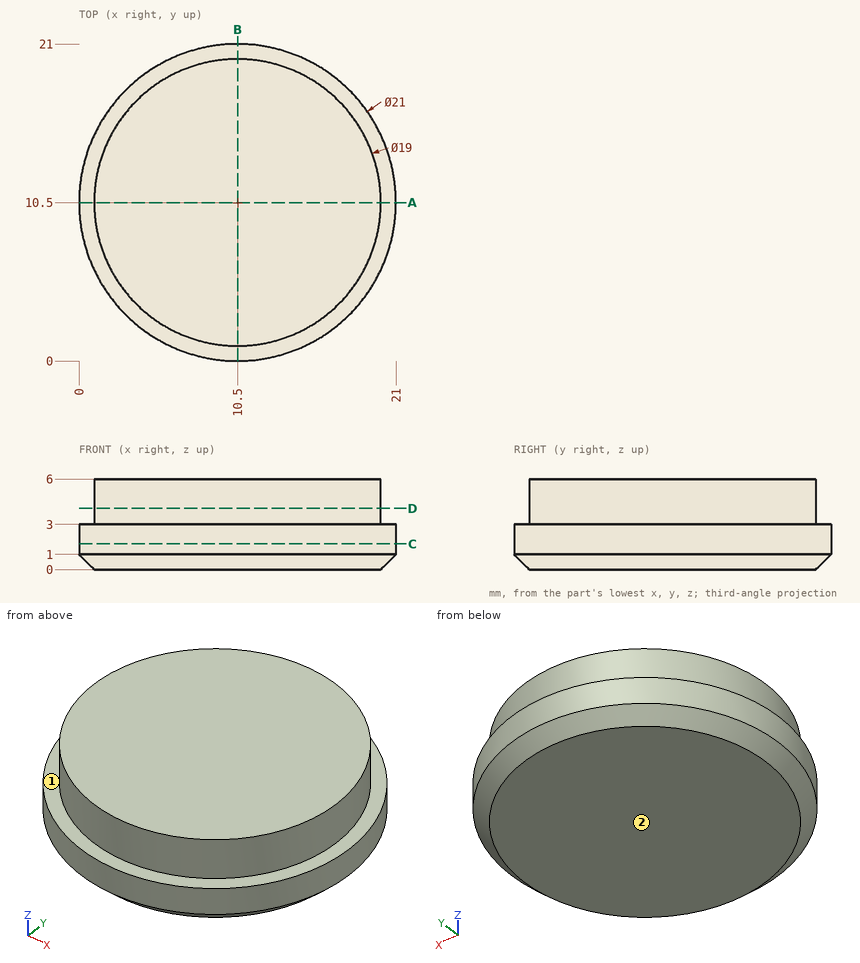
Verification items for this drawing (mm, ordinates from the low corner). A direction names the side the tool comes from. Coordinates: 2 decimals unless noted, no trailing zeros. Write each loop counter-clockwise with the first axis right and the second up, starting at its lowest first coordinate (ties: lowest second). Pieces come first, ordered by that corner, then holes. Notation, with made-up numbers: M 77.25,5 L 100.25,5 A28 ccw 100.25,33 Z; hole C -25,-26.5 d1. An arc over 180 degrees is marked long. One line per item, written item: value. Start each with the question number.
(1) Sectioned sample at C-C, the plane z = 1.7. Enter the section's corners in (x, y).
(2) Scan lines: line 1 along Y through (x, z) = (17.75, 5.55); line 2 along Y through (x, z) = (8.5, 5.4); line 3 along Z through (x, y) = (1.5, 6). Record each from-to range of solid material in increasing order. Write a range as [from, to].
(3) Sectioned sample at D-D, the plane z = 4.05. Enter the section's corners in (x, y).
(4) Sectioned sample at A-A, the plane y = 10.5. Enter the section's corners in (x, z), and give its area (3 significant figures).
(5) Tool access check on the marked faces 1 and 2. Record the directions out of +Z, -Z, +X, -X, +Y, -Y that give a thin tool (end or side, any length) a straight path to the whole face; none if there is none.
Filled sheet:
1. outline: C 10.5,10.5 d21
2. line 1: [4.36, 16.64]
2. line 2: [1.21, 19.79]
2. line 3: [0.56, 3]
3. outline: C 10.5,10.5 d19
4. outline: M 0,1 L 1,0 L 20,0 L 21,1 L 21,3 L 20,3 L 20,6 L 1,6 L 1,3 L 0,3 Z
4. area: 119 mm²
5. face 1: +Z
5. face 2: -Z, +X, -X, +Y, -Y
